```python
from build123d import *

# Parameters (mm, degrees)
CYLINDER_R      = 11.5
CYLINDER_DEPTH  = 2
SKETCH002_W     = 6
SKETCH002_H     = 6
PAD001_DEPTH    = 1
SKETCH003_R     = 2
POCKET001_DEPTH = 1
SKETCH004_W     = 6
SKETCH004_H     = 6
PAD002_DEPTH    = 1
SKETCH005_R     = 2
POCKET002_DEPTH = 1


with BuildPart() as part:
    # Cylinder → Cylinder (new body)
    with BuildSketch(Plane.XY):
        Circle(CYLINDER_R)
    extrude(amount=CYLINDER_DEPTH)

    # Sketch002 → Pad001 (new body)
    with BuildSketch(Plane.XY.offset(2)):
        Rectangle(SKETCH002_W, SKETCH002_H)
    extrude(amount=PAD001_DEPTH)

    # Sketch003 → Pocket001 (cut)
    with BuildSketch(Plane.XY.offset(3)):
        Circle(SKETCH003_R)
    extrude(amount=-POCKET001_DEPTH, mode=Mode.SUBTRACT)

    # Sketch004 → Pad002 (new body)
    with BuildSketch(Plane.XY.offset(2)):
        with Locations((0, 6.7)):
            Rectangle(SKETCH004_W, SKETCH004_H)
        with Locations((-6.7, 0)):
            Rectangle(SKETCH004_W, SKETCH004_H)
        with Locations((0, -6.7)):
            Rectangle(SKETCH004_W, SKETCH004_H)
        with Locations((6.7, 0)):
            Rectangle(SKETCH004_W, SKETCH004_H)
    extrude(amount=PAD002_DEPTH)

    # Sketch005 → Pocket002 (cut)
    with BuildSketch(Plane.XY.offset(3)):
        with Locations((0, 6.615592)):
            Circle(SKETCH005_R)
        with Locations((-6.615583, 0)):
            Circle(SKETCH005_R)
        with Locations((6.712149, 0)):
            Circle(SKETCH005_R)
        with Locations((0, -6.712142)):
            Circle(SKETCH005_R)
    extrude(amount=-POCKET002_DEPTH, mode=Mode.SUBTRACT)


with BuildPart() as part_1:
    # Clone001 placement: moved
    add(part.part.moved(Location((-7, -6, -13))))


solid = part_1.part
```
Work out the finished part from the listing and answer in its coordinate system (mm). A direction names the side the tool comes from. Give positions to 0.01 mm unless a question says otherwise; leave off trailing zeros. Loops run counter-clockwise (first coordinate to the right, second up) from the corner with the lowest first, then second, coordinate; pieces in that order, holes last. Notation, with made-up numbers: (69.5, -26) -> (116.5, -26) arc R19 ccw to (116.5, 6) -> close; hole circle Ø5 at (59.5, 6.5). An arc over 180 degrees is marked (long way). Write item = value, one per line. Start each with the question number.
(1) Find section B-B on x = -7. Give the vertices of the cut face in (y, z).
(2) Find section D-D on x = -13.75. Give the vertices of the cut face in (y, z).
(3) Find section A-A on y = -6. Give the vertices of the cut face in (x, z).
(4) Find section C-C on z = -12.6. Give the vertices of the cut face in (x, y).
(5) The mould has two halves that part along Y. Classify faces 4 (the flat face through (-0.3, -3, -10.5)), 5 (the flat face through (-2.34, -5.29, -10)), 6 (the flat face through (-7, -2.3, -10.5)): +Y half, -Y half, draft (parallel to the pull), parting line (faces both ways), or undercut.
(6) Find the intervals of material crossed by probe 1 along Y at (x, z) = (-7, -10.75); probe 2 along X at (y, z) = (-8.5, -10.75); probe 3 along Y at (x, z) = (-13.5, -10.65), in increasing order. Write a range as from..to.
(7) Given pin 1 Ø0.8 at (y, z) = (-6, -10.5) entering from -X; pin 2 Ø1.5 at (x, y) = (-11.5, 0.5) entering from +Z; pin 3 Ø4.5 at (x, y) = (-12.5, -6.5) entering from +Z; pin 4 Ø1.5 at (x, z) = (-10.5, -11) entering from -Y, each flat-ended and moving along its own axis, determine where each tip first touches the part or whether it passes through.
(8) Which of the six approach directions +Z, -Z, +X, -X, +Y, -Y give full straight-line access (tool end or side, diameter ignored) to faces 1 (the flat face through (-7, -6, -11)), 2 (the flat face through (-7, -3, -10.5)), 3 (the flat face through (-0.3, -9, -10.5))?
From the geometry:
q1.outline = (-17.5, -13) -> (5.5, -13) -> (5.5, -11) -> (3.7, -11) -> (3.7, -10) -> (2.62, -10) -> (2.62, -11) -> (-1.38, -11) -> (-1.38, -10) -> (-2.3, -10) -> (-2.3, -11) -> (-3, -11) -> (-3, -10) -> (-4, -10) -> (-4, -11) -> (-8, -11) -> (-8, -10) -> (-9, -10) -> (-9, -11) -> (-9.7, -11) -> (-9.7, -10) -> (-10.71, -10) -> (-10.71, -11) -> (-14.71, -11) -> (-14.71, -10) -> (-15.7, -10) -> (-15.7, -11) -> (-17.5, -11) -> close
q2.outline = (-15.31, -13) -> (3.31, -13) -> (3.31, -11) -> (-3, -11) -> (-3, -10) -> (-4, -10) -> (-4, -11) -> (-8, -11) -> (-8, -10) -> (-9, -10) -> (-9, -11) -> (-15.31, -11) -> close
q3.outline = (-18.5, -13) -> (4.5, -13) -> (4.5, -11) -> (2.7, -11) -> (2.7, -10) -> (1.71, -10) -> (1.71, -11) -> (-2.29, -11) -> (-2.29, -10) -> (-3.3, -10) -> (-3.3, -11) -> (-4, -11) -> (-4, -10) -> (-5, -10) -> (-5, -11) -> (-9, -11) -> (-9, -10) -> (-10, -10) -> (-10, -11) -> (-10.7, -11) -> (-10.7, -10) -> (-11.62, -10) -> (-11.62, -11) -> (-15.62, -11) -> (-15.62, -10) -> (-16.7, -10) -> (-16.7, -11) -> (-18.5, -11) -> close
q4.outline = circle Ø23 at (-7, -6)
q5.face_4 = +Y half
q5.face_5 = draft
q5.face_6 = undercut
q6.probe_1 = -15.7..-14.71, -10.71..-9.7, -9..-8, -4..-3, -2.3..-1.38, 2.62..3.7
q6.probe_2 = -16.7..-10.7, -10..-4, -3.3..2.7
q6.probe_3 = -9..-8, -4..-3
q7.pin_1 = -16.7
q7.pin_2 = -11
q7.pin_3 = -10
q7.pin_4 = -17.17
q8.face_1 = +Z
q8.face_2 = +Z, +X, -X
q8.face_3 = +Z, +X, -X, -Y
